Design review of the part built by this model. Coordinates are the model's own, in mm. Face numbers are marked on the shaded views. A direction names the side the tool comes from. Give positions to 0.01 mm unless a question says otherwise; leave off trailing zeros. Loops run counter-clockwise (first coordinate to the right, second up) from the corner with the lowest first, then second, coordinate; pieces in that order, holes last. Notation, with made-up numbers: (-39.75, 37.5) -> (6.25, 37.5) arc R26 cw to (6.25, 62.5) -> close; hole circle Ø10 at (30, 51). An arc over 180 degrees is marked (long way). Answer in a Markdown table with one row per item. Add a question column.
(1) Draft analysis for pull direction Z (two halves, no side actions). For the marked faces 1, 2, 3 and 4, state which applies: +Z half, -Z half, draft (parallel to the pull), parting line (faces both ways), or undercut.
(2) For the marked faces 5, 6, 7, 8 and 9, list the 3-axis set-ups (+Z, -Z, +X, -X, +Y, -Y) from which the entire face can be reached by the end or side of a thin tool; tool diameter is ignored.
(3) Consider section A-A on y = -0.5. Write out the cut boundary in (x, z).
(4) For line 1 (Z direction, x = 0, y = 1); line 2 (Y direction, x = 4, z = 5); line 3 (X direction, y = 2.75, z = 1.5), list the stretches that pass through material, from the lowest coordinate up.
(5) Consider section B-B on y = 3.5. Write out the cut boundary in (x, z), then the cut area to 3 significant figures.
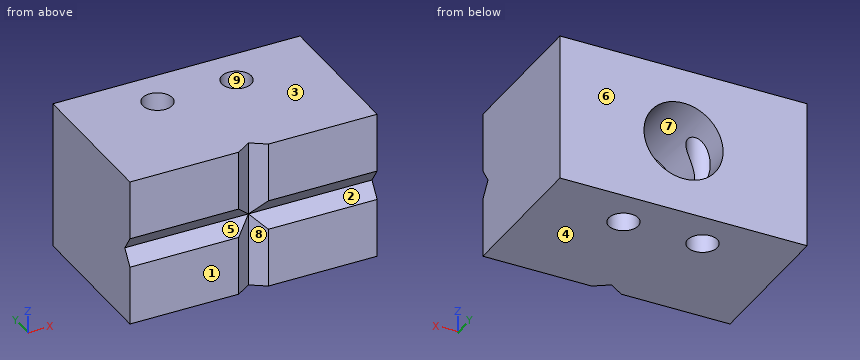
from build123d import *

# Parameters (mm, degrees)
SKETCH1_W                 = 25
SKETCH1_H                 = 15
BOSS_EXTRUDE1_DEPTH       = 15
F_3_0MM_DOWEL_HOLE1_D     = 3
CUT_EXTRUDE1_DEPTH        = 15
CUT_EXTRUDE2_DEPTH        = 49
F_8_0MM_DOWEL_HOLE1_D     = 8
F_8_0MM_DOWEL_HOLE1_DEPTH = 9
F_8_0MM_DOWEL_HOLE1_TIP   = 2.403442476


with BuildPart() as part:
    # Sketch1 → Boss-Extrude1 (new body)
    with BuildSketch(Plane.XY):
        Rectangle(SKETCH1_W, SKETCH1_H)
    extrude(amount=BOSS_EXTRUDE1_DEPTH)

    # Ø3.0mm Dowel Hole1 (through all)
    with Locations(Plane(origin=(0, 0, 0), x_dir=(-1, 0, 0), z_dir=(0, 0, -1))):
        with Locations((4, 3.5), (-4, 3.5)):
            Hole(F_3_0MM_DOWEL_HOLE1_D / 2)

    # Sketch4 → Cut-Extrude1 (cut)
    with BuildSketch(Plane(origin=(0, 0, 0), x_dir=(-1, 0, 0), z_dir=(0, 0, -1))):
        Polygon((-1.5, -7.5), (0, -6.5), (1.5, -7.5), (1.5, -8.661877418), (-1.5, -8.661877418), align=None)
    extrude(amount=-CUT_EXTRUDE1_DEPTH, mode=Mode.SUBTRACT)

    # Sketch5 → Cut-Extrude2 (cut)
    with BuildSketch(Plane.ZY.offset(12.5)):
        Polygon((6, -7.5), (7.5, -6.5), (9, -7.5), (9, -8.497485746), (6.14045431, -8.497485746), align=None)
    extrude(amount=-CUT_EXTRUDE2_DEPTH, mode=Mode.SUBTRACT)

    # Ø8.0mm Dowel Hole1
    with Locations(Plane(origin=(0, 7.5, 0), x_dir=(1, 0, 0), z_dir=(0, 1, 0))):
        with Locations((0, -7.5)):
            Hole(F_8_0MM_DOWEL_HOLE1_D / 2, depth=F_8_0MM_DOWEL_HOLE1_DEPTH)
            with Locations((0, 0, -(F_8_0MM_DOWEL_HOLE1_DEPTH + F_8_0MM_DOWEL_HOLE1_TIP / 2))):  # 118° drill point
                Cone(0, F_8_0MM_DOWEL_HOLE1_D / 2, F_8_0MM_DOWEL_HOLE1_TIP, mode=Mode.SUBTRACT)


solid = part.part
Values follow:
| question | item | result |
|---|---|---|
| 1 | face 1 | draft |
| 1 | face 2 | undercut |
| 1 | face 3 | +Z half |
| 1 | face 4 | -Z half |
| 2 | face 5 | +X, -X, -Y |
| 2 | face 6 | +Z, -Z, +X, -X, +Y |
| 2 | face 7 | +Y |
| 2 | face 8 | +Z, -Z, -Y |
| 2 | face 9 | +Z, -Z |
| 3 | outline | (-12.5, 0) -> (12.5, 0) -> (12.5, 15) -> (-12.5, 15) -> close; hole circle Ø8 at (0, 7.5) |
| 4 | line 1 | 0 to 3.5, 11.5 to 15 |
| 4 | line 2 | -7.5 to 2, 5 to 7.5 |
| 4 | line 3 | -12.5 to -5.3, -2.7 to 2.7, 5.3 to 12.5 |
| 5 | outline | (-12.5, 0) -> (-5.5, 0) -> (-5.5, 15) -> (-12.5, 15) -> close; (-2.5, 0) -> (2.5, 0) -> (2.5, 4.38) arc R4 cw to (-2.5, 4.38) -> close; (-2.5, 10.62) arc R4 cw to (2.5, 10.62) -> (2.5, 15) -> (-2.5, 15) -> close; (5.5, 0) -> (12.5, 0) -> (12.5, 15) -> (5.5, 15) -> close |
| 5 | area | 248 mm2 |
